Model file for the job. Use its own axes, mm. A direction names the side the tool comes from. Give positions to 0.01 mm unless a question says otherwise; leave off trailing zeros. Loops run counter-clockwise (first coordinate to the right, second up) from the corner with the lowest first, then second, coordinate; pieces in that order, holes last. Notation, with made-up numbers: M 85.25,76 L 124.25,76 A12 ccw 124.25,94 Z; hole C 40,19 d9. An arc over 180 degrees is marked long. Use CSV: the item, a comma, the result in double quotes. Start each with the question number.
(1) Tool access for faces 1 (the face through (5.05, 2.5, 0.1)), 2 (the face through (1, 6, -11.35)), 3 (the face through (1, 6, 11.35)), 4 (the face through (0, 6, 9.85)), 5 (the face through (3.15, 2.24, -5.903)): list every direction of +Z, -Z, +X, -X, +Y, -Y with a clear straight run to the whole face (end or side of a thin tool).
(2) Slice it at A-A on z = 4.75. List the corners of the cut face in (x, y).
(3) Slice it at C-C on z = 0.5. List the corners of the cut face in (x, y).
(4) Two-plate mould, pull along Z, no slides. Class faces 6 (the face through (-3.55, 1.48, 14.27)), 7 (the face through (3.15, 2.24, 3.597)), 8 (the face through (1, 10, 11)): pulls with the +Z half, pulls with the -Z half, needs draft (parallel to the pull), parting line crosses it, or undercut.
(5) Wall check: line 1 along Z through (x, y) = (0, 1.95); line 2 along Z through (x, y) = (5.5, 4.5); line 3 along Z through (x, y) = (2.55, 2.6). Give the ranges that are in metal, low to high. Write a range as from..to.
(6) Slice it at B-B on y = 8.25. List the corners of the cut face in (x, z), and give its area (3 significant figures).
(7) Flat gauge pins, fed straight in: P1, Ø3, axis at x = 5.5, y = 6.5, coming from the -Z side; P2, Ø4, axis at x = 3, y = 1.5, coming from the +Z side; P3, Ø2, axis at x = 6, y = 5, coming from the +Z side; P4, Ø5, axis at x = -1, y = 5, coming from the -Z side. Where does each tip first touch, or does it go through?
(8) Slice it at D-D on x = 3. State how many separate pieces and enclosed holes the cut face has, and give its area (3 significant figures).
Autodesk Inventor part; units mm, degrees
ref_plane "YZ Plane" through (0, 0, 0) normal (1, 0, 0) x (0, 1, 0)
ref_plane "XZ Plane" through (0, 0, 0) normal (0, 1, 0) x (-1, 0, 0)
ref_plane "XY Plane" through (0, 0, 0) normal (0, 0, 1) x (1, 0, 0)
sketch "Эскиз1" plane through (0, 0, 0) normal (0, 1, 0) x (-1, 0, 0)
  line L0 (5.05, 9.85) -> (-5.05, 9.85)
  line L1 (-5.05, 9.85) -> (-5.05, -9.85)
  line L2 (-5.05, -9.85) -> (5.05, -9.85)
  line L3 (5.05, -9.85) -> (5.05, 9.85)
  line L4 (5.05, 9.85) -> (-5.05, -9.85) construction
  line L5 (-5.05, 9.85) -> (5.05, -9.85) construction
  line L6 (7.05, -11.35) -> (5.05, -11.35) construction
  line L7 (-7.05, -11.35) -> (-7.05, 11.35)
  line L8 (-7.05, 11.35) -> (5.05, 11.35)
  line L9 (7.05, 11.35) -> (7.05, -11.35) construction
  line L10 (5.05, 9.85) -> (5.05, 11.35)
  line L11 (5.05, -9.85) -> (5.05, -11.35)
  line L12 (5.05, 11.35) -> (7.05, 11.35) construction
  line L13 (5.05, -11.35) -> (-7.05, -11.35)
  point P0 (0, 0)
  dimension "d0" = 10.1
  dimension "d1" = 19.7
  dimension "d2" = 1.5
  dimension "d24" = 1.5
extrude "Выдавливание1" add sketch "Эскиз1" along normal blind 10 contours L0 L1 L2 L11 L13 L7 L8 L10
sketch "Эскиз2" plane through (0, 0, 0) normal (0, -1, 0) x (1, 0, 0)
  line L0 (-5.05, 11.35) -> (7.05, 11.35)
  line L1 (7.05, 11.35) -> (-5.05, 11.35)
  line L2 (-5.05, 11.35) -> (-5.05, -11.35)
  line L3 (-5.05, -11.35) -> (7.05, -11.35)
  line L4 (7.05, -11.35) -> (7.05, 11.35)
  line L5 (0, 16.25) -> (0, -16.25)
  circle A0 centre (0, 16.25) radius 2.25
  circle A1 centre (0, -16.25) radius 2.25
  line L6 (1.7234, 17.6965) -> (7.05, 11.35)
  line L7 (-5.05, 11.35) -> (-2.0009, 17.279)
  line L8 (7.05, -11.35) -> (-5.05, -11.35)
  line L9 (7.05, -11.35) -> (1.7234, -17.6965)
  line L10 (-5.05, -11.35) -> (-2.0009, -17.279)
  circle A2 centre (0, 16.25) radius 1.6
  circle A3 centre (0, -16.25) radius 1.6
  circle A4 centre (2.55, -4.75) radius 1.3
  circle A5 centre (2.55, 4.75) radius 1.3
  line L11 (5.05, -9.85) -> (5.05, 9.85)
  line L12 (2.55, -4.75) -> (2.55, 4.75)
  line L13 (0, 0) -> (7.05, 0)
  line L14 (7.05, 11.35) -> (7.05, -11.35)
  point P0 (-5.05, 11.35)
  point P1 (2.55, 0)
  point P2 (-5.05, 11.35)
  dimension "d5" = 32.5
  dimension "d6" = 4.5
  dimension "d10" = 4.5
  dimension "d12" = 3.2
  dimension "d13" = 3.2
  dimension "d16" = 2.6
  dimension "d17" = 2.6
  dimension "d18" = 2.5
  dimension "d19" = 2.5
  dimension "d20" = 9.5
extrude "Выдавливание2" add sketch "Эскиз2" against normal blind 3
chamfer "Фаска1" distance 1.5 angle 45 2 edges at (1.25, 0, -4.75) (1.25, 0, 4.75)
sketch "Эскиз3" plane through (7.05, 10, 11.35) normal (1, 0, 0) x (0, 0, -1)
  line L0 (22.7, -7) -> (22.7, 0)
  line L1 (0, 0) -> (22.7, 0)
  line L2 (0, -7) -> (0, 0)
  line L3 (0, -10) -> (0, -7)
  line L4 (0, -10) -> (22.7, -10)
  line L5 (22.7, -10) -> (22.7, -7)
  line L6 (20.7, -2) -> (20.7, -7)
  line L7 (20.7, -7) -> (20.7, -8)
  line L8 (20.7, -8) -> (2, -8)
  line L9 (2, -8) -> (2, -7)
  line L10 (2, -7) -> (2, -2)
  line L11 (2, -2) -> (20.7, -2)
  line L12 (20.7, -2) -> (20.7, 0)
  line L13 (0, 0) -> (22.7, 0)
  line L14 (2, -2) -> (2, 0)
  point P0 (11.35, -10)
  dimension "d25" = 2
extrude "Выдавливание3" cut sketch "Эскиз3" against normal blind 2 contours L12 L11 L14 L1 | L6 L7 L8 L9 L10 L11
properties part number "креп_концевика"
Reply:
1,face 1,"+X, +Y"
1,face 2,"-Z, +X, -X, +Y"
1,face 3,"+Z, +X, -X, +Y"
1,face 4,"-X, +Y"
1,face 5,"+Y, -Y"
2,outline,"M -5.05,0 L -0.25,0 L 1.25,1.5 L 1.25,3 L -5.05,3 Z; M 3.85,1.5 L 5.35,0 L 7.05,0 L 7.05,2 L 5.05,2 L 5.05,3 L 3.85,3 Z"
3,outline,"M -5.05,0 L 7.05,0 L 7.05,2 L 5.05,2 L 5.05,3 L -5.05,3 Z"
4,face 6,"pulls with the +Z half"
4,face 7,"undercut"
4,face 8,"needs draft"
5,line 1,"z = -18.5..-17.85, -14.65..14.65, 17.85..18.5"
5,line 2,"z = -11.35..-9.35, 9.35..11.35"
5,line 3,"z = -16.71..-6.05, -3.45..3.45, 6.05..16.71"
6,outline,"M -5.05,-11.35 L 7.05,-11.35 L 7.05,-9.35 L 5.05,-9.35 L 5.05,-9.85 L -5.05,-9.85 Z; M -5.05,9.85 L 5.05,9.85 L 5.05,9.35 L 7.05,9.35 L 7.05,11.35 L -5.05,11.35 Z"
6,area,"38.3 mm^2"
7,P1,"stops at z = -11.35"
7,P2,"stops at z = 18.27"
7,P3,"stops at z = 11.35"
7,P4,"stops at z = -18.5"
8,separate pieces,"3"
8,enclosed holes,"0"
8,area,"98.8 mm^2"
